Could you check a few things on this model? Use its own coordinates, in mm. Face numbers are marked on the shaded views. A direction names the side the tool comes from. Give positions to 0.01 mm unless a question says otherwise; leave off trailing zeros. Order: outer loops, then holes, each group sorted by start corner. A loop starts at its lowest first (then second) coordinate and runs counter-clockwise, first axis right, second up.
(1) Imagine slicing it at C-C, the plane x = -16.25. State how many separate pieces and enclosed holes the cut face has, then the cut area to 3 significant figures.
(2) If I drill on probe 1 along Z at (x, y) = (-5.25, 0) (3 decimals); probe 2 along Y at (x, z) = (-12.25, 9); probe 3 along Z at (x, y) = (-11.75, 6) (3 decimals), over which ranges is the centre line in solid material (lowest first)?
(3) On a 3-axis mill with a long thin cutter (end or side, diameter ignored), from which of +Z, -Z, +X, -X, +Y, -Y can I reach the whole of each face in a straight line? I mean the marked faces 4, 5 and 6. Say none if no direction works.
(4) Imagine slicing it at A-A, the plane z = 16.5. Write out the boundary of the cut face in (x, y) (3 decimals), then the cut area to 3 significant figures.
(5) Imagine slicing it at D-D, the plane y = 17.5. Write out the boundary of the cut face in (x, z) (3 decimals).
(6) Imagine slicing it at B-B, the plane y = 0. Write out the boundary of the cut face in (x, z) (3 decimals).
(7) Will these pins go through, and if not, where does the flat tip stop? pin 1 (8.5 mm diameter, centred on x = -9.525, y = 9.525, fed in from -Z); pin 2 (1 mm diameter, centred on x = -3, z = -16.5, fed in from +Y); pin 3 (1.9 mm diameter, centred on x = -6, z = 9, fed in from +Y).
(8) If we mould it in two halves opening along Y, with no side actions, what happens to the marked faces 1, 2 and 3? For each: released by +Y, released by -Y, zero draft, split by the parting line, or undercut.
Autodesk Inventor part; units mm, degrees
ref_plane "YZ Plane" through (0, 0, 0) normal (1, 0, 0) x (0, 1, 0)
ref_plane "XZ Plane" through (0, 0, 0) normal (0, 1, 0) x (-1, 0, 0)
ref_plane "XY Plane" through (0, 0, 0) normal (0, 0, 1) x (1, 0, 0)
sketch "Sketch1" plane through (0, 0, 0) normal (1, 0, 0) x (0, 1, 0)
  line L0 (19.05, 22.225) -> (-19.05, 22.225)
  line L1 (-19.05, 22.225) -> (-19.05, -22.225)
  line L2 (-19.05, -22.225) -> (19.05, -22.225)
  line L3 (19.05, -22.225) -> (19.05, 22.225)
  line L4 (19.05, 22.225) -> (-19.05, -22.225) construction
  line L5 (-19.05, 22.225) -> (19.05, -22.225) construction
  line L6 (19.05, -15.875) -> (1.5875, -15.875)
  line L7 (1.5875, -15.875) -> (1.5875, 3.175)
  line L8 (1.5875, 3.175) -> (19.05, 3.175)
  line L9 (19.05, 3.175) -> (19.05, -15.875)
  line L10 (-19.05, 17.4625) -> (19.05, 17.4625) construction
  point P0 (0, 0)
  point P1 (-12.7, 17.4625)
  point P2 (0, 17.4625)
  point P3 (-12.7, 7.9375)
  point P4 (0, 7.9375)
  dimension "d0" = 38.1
  dimension "d1" = 44.45
  dimension "d2" = 17.4625
  dimension "d3" = 19.05
  dimension "d4" = 6.35
  dimension "d31" = 4.7625
  dimension "d32" = 6.35
  dimension "d35" = 12.7
  dimension "d38" = 9.525
extrude "Extrusion1" add sketch "Sketch1" against normal blind 19.05 contours L3 L8 L7 L6 L2 L1 L0
sketch "Sketch2" plane through (0, -19.05, -22.225) normal (0, 0, -1) x (-1, 0, 0)
  line L0 (0, 38.1) -> (19.05, 38.1)
  line L1 (0, 0) -> (0, 38.1)
  point P0 (0, 19.05)
  point P1 (9.525, 28.575)
  dimension "d7" = 9.525
  dimension "d8" = 9.525
hole "Hole1" at (-9.525, 9.525, -22.225) direction (0, 0, 1) diameter 6.35 end through all counterbore diameter 9.525 counterbore depth 3.175
sketch "Sketch3" plane through (-19.05, 0, 0) normal (-1, 0, 0) x (0, 0, 1)
  line L0 (3.175, 6.35) -> (3.175, 12.7)
  line L1 (22.225, 12.7) -> (22.225, 6.35)
  line L2 (3.175, 6.35) -> (3.175, 12.7)
  line L3 (3.175, 19.05) -> (3.175, 1.5875)
  line L4 (3.175, 9.525) -> (22.225, 9.525) construction
  line L5 (22.225, -19.05) -> (22.225, 19.05)
  line L6 (22.225, 19.05) -> (3.175, 19.05)
  line L7 (12.7, 14.2875) -> (6.35, 14.2875)
  line L8 (6.35, 14.2875) -> (6.35, 4.7625)
  line L9 (6.35, 4.7625) -> (12.7, 4.7625)
  line L10 (12.7, 4.7625) -> (12.7, 14.2875)
  line L11 (12.7, 14.2875) -> (6.35, 4.7625) construction
  line L12 (6.35, 14.2875) -> (12.7, 4.7625) construction
  point P0 (0, 0)
  point P1 (9.525, 9.525)
  dimension "d16" = 9.525
  dimension "d17" = 6.35
  dimension "d18" = 9.525
  dimension "d19" = 3.175
extrude "Extrusion2" cut sketch "Sketch3" against normal through all
fillet "Fillet1" radius 9.525 6 edges at (0, 19.05, 12.7) (0, 19.05, -19.05) (-19.05, 19.05, -19.05) (-19.05, 19.05, 12.7) (-19.05, 1.5875, -6.35) (0, 1.5875, -6.35)
chamfer "Chamfer1" distance 12.7 angle 45 1 edges at (-9.525, -19.05, -22.225)
fillet "Fillet2" radius 9.525 2 edges at (-9.525, -6.35, -22.225) (-9.525, -19.05, -9.525)
thicken "Thicken1" operation add thickness 0.1 both sides no extend neighbours yes toward (0, 0, 1) faces at (-3.6754, 5.7159, 3.175)
thicken "Thicken2" operation add thickness 0.1 both sides no extend neighbours yes toward (0, 0, -1) faces at (-3.6754, 5.7159, -15.875)
hole "Hole2" at (0, -12.7, 17.4625) at (0, 0, 17.4625) at (0, -12.7, 7.9375) at (0, 0, 7.9375) direction (-1, 0, 0) diameter 3.175 end through all
sketch "Sketch4" plane through (-19.05, 0, 0) normal (-1, 0, 0) x (0, 0, 1)
  point P0 (17.4625, 0)
  point P1 (7.9375, 0)
  point P2 (7.9375, -12.7)
  point P3 (17.4625, -12.7)
  point P4 (93.6625, -12.7)
  point P5 (84.1375, -12.7)
  point P6 (84.1375, 0)
  point P7 (93.6625, 0)
hole "Hole3" at (-19.05, 0, 17.4625) at (-19.05, 0, 7.9375) at (-19.05, -12.7, 7.9375) at (-19.05, -12.7, 17.4625) at (-19.05, -12.7, 93.6625) at (-19.05, -12.7, 84.1375) at (-19.05, 0, 84.1375) at (-19.05, 0, 93.6625) direction (1, 0, 0) diameter 3.7973 depth 19.05
properties part number "Side Mounts" material "Nylon 6/6"
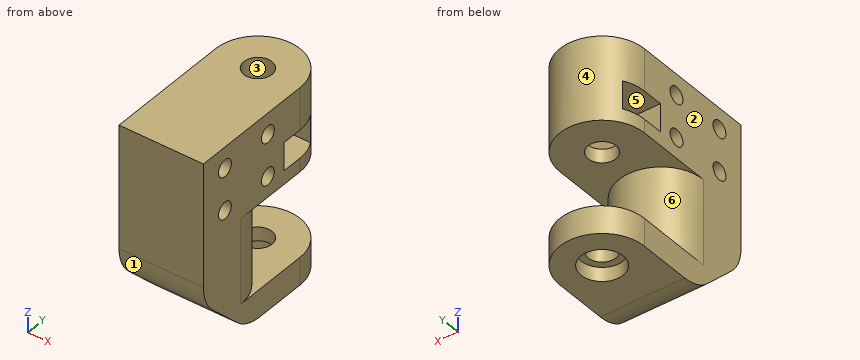
Answer block:
1. separate pieces: 1
1. enclosed holes: 5
1. area: 1,040 mm2
2. probe 1: z = -22.225 to 6.039, 9.836 to 15.564, 19.361 to 22.225
2. probe 2: y = -19.05 to -14.27, -11.13 to -1.57, 1.57 to 4.76, 14.29 to 18.65
2. probe 3: z = -19.05 to -15.975, 3.275 to 6.35, 12.7 to 22.225
3. face 4: +Z, -Z, +Y
3. face 5: +X, -X
3. face 6: +Y
4. outline: (-19.05, -19.05) - (0, -19.05) - (0, -14.337) - (-19.05, -14.337) - close; (-19.05, -11.063) - (0, -11.063) - (0, -1.637) - (-19.05, -1.637) - close; (-19.05, 1.637) - (0, 1.637) - (0, 9.525) arc R9.525 ccw to (-19.05, 9.525) - close; hole circle Ø6.35 at (-9.525, 9.525)
4. area: 530 mm2
5. outline: (-14.733, -22.225) - (-4.317, -22.225) - (-4.317, -15.975) - (-14.733, -15.975) - close; (-14.733, 3.275) - (-4.317, 3.275) - (-4.317, 22.225) - (-14.733, 22.225) - close
6. outline: (-19.05, -22.225) - (0, -22.225) - (0, -15.975) - (-4.26, -15.975) - (-4.26, 3.275) - (0, 3.275) - (0, 6.039) - (-19.05, 6.039) - (-19.05, 3.275) - (-14.79, 3.275) - (-14.79, -15.975) - (-19.05, -15.975) - close; (-19.05, 9.836) - (0, 9.836) - (0, 15.564) - (-19.05, 15.564) - close; (-19.05, 19.361) - (0, 19.361) - (0, 22.225) - (-19.05, 22.225) - close
7. pin 1: stops at z = -19.05
7. pin 2: stops at y = 16.9
7. pin 3: stops at y = 18.7
8. face 1: released by -Y
8. face 2: zero draft
8. face 3: undercut
